```python
from build123d import *

# Parameters (mm, degrees)
F2_DEPTH = 10.16
F3_R     = 2.413
F4_DEPTH = 10.16
F5_R     = 5.08
F6_R     = 1.27
F8_DEPTH = 10.16
F9_R     = 5.08


# Not quite as in the source:
# - a variable given as a bare number and used for a length is read in inches; the dataset says mm whatever the document's units were
# - a feature names something its author has since deleted; it is built from what else it names


with BuildPart() as f2:
    # F1 (on Top) → F2 (new body)
    with BuildSketch(Plane.XY):
        with BuildLine():
            Line((0, 0), (0, -76.2))
            Line((0, -76.2), (0, -82.55))
            ThreePointArc((0, -82.55), (4.4901280605, -80.6901280605), (6.35, -76.2))
            Line((6.35, -76.2), (6.35, 5.1130828846))
            ThreePointArc((6.35, 5.1130828846), (-16.8661271179, 9.1115403998), (-40.386, 10.4501219109))
            ThreePointArc((-40.386, 10.4501219109), (-63.9058728821, 9.1115403998), (-87.122, 5.1130828846))
            Line((-87.122, 5.1130828846), (-87.122, -76.2))
            ThreePointArc((-87.122, -76.2), (-85.2621280605, -80.6901280605), (-80.772, -82.55))
            Line((-80.772, -82.55), (-80.772, -76.2))
            Line((-80.772, -76.2), (-80.772, 0))
            ThreePointArc((-80.772, 0), (-60.6827977504, 3.072463713), (-40.386, 4.1001219109))
            ThreePointArc((-40.386, 4.1001219109), (-20.0892022496, 3.072463713), (0, 0))
        make_face()
    extrude(amount=F2_DEPTH)

    # F3 (on Top) → F4 (join)
    with BuildSketch(Plane.XY):
        with Locations((0, -7.9375)):
            Circle(F3_R)
        with Locations((-80.772, -7.9375)):
            Circle(F3_R)
    extrude(amount=F4_DEPTH)

    # F5
    f5_edges = [f2.edges().sort_by_distance(p)[0] for p in [
        (-87.122, 5.113083, 5.08),
        (6.35, 5.113083, 5.08),
    ]]
    fillet(f5_edges, radius=F5_R)

    # F6
    f6_edges = [f2.edges().sort_by_distance(p)[0] for p in [
        (0, -82.55, 5.08),
        (-80.772, -82.55, 5.08),
        (0, 0, 5.08),
        (-80.772, 0, 5.08),
    ]]
    fillet(f6_edges, radius=F6_R)

    # F7 (on Top) → F8 (join)
    with BuildSketch(Plane.XY):
        with BuildLine():
            ThreePointArc((31.75, -25.4), (19.05, -38.1), (6.35, -25.4))
            Line((6.35, -25.4), (6.35, -65.42595876))
            ThreePointArc((6.35, -65.42595876), (11.6697145424, -58.7651555547), (19.05, -54.499355663))
            ThreePointArc((19.05, -54.499355663), (32.9139558425, -42.7901912008), (38.1, -25.4))
            ThreePointArc((38.1, -25.4), (34.925, -28.575), (31.75, -25.4))
        make_face()
        with BuildLine():
            ThreePointArc((38.1, -25.4), (34.925, -22.225), (31.75, -25.4))
            ThreePointArc((31.75, -25.4), (34.925, -28.575), (38.1, -25.4))
        make_face()
        with BuildLine():
            Line((-87.122, -65.42595876), (-87.122, -25.4))
            ThreePointArc((-87.122, -25.4), (-99.822, -38.1), (-112.522, -25.4))
            ThreePointArc((-112.522, -25.4), (-115.697, -28.575), (-118.872, -25.4))
            ThreePointArc((-118.872, -25.4), (-113.6859558425, -42.7901912008), (-99.822, -54.499355663))
            ThreePointArc((-99.822, -54.499355663), (-92.4417145424, -58.7651555547), (-87.122, -65.42595876))
        make_face()
        with BuildLine():
            ThreePointArc((-118.872, -25.4), (-115.697, -28.575), (-112.522, -25.4))
            ThreePointArc((-112.522, -25.4), (-115.697, -22.225), (-118.872, -25.4))
        make_face()
    extrude(amount=F8_DEPTH)

    # F9
    f9_edges = [f2.edges().sort_by_distance(p)[0] for p in [
        (6.35, -65.425959, 5.08),
        (-87.122, -65.425959, 5.08),
    ]]
    fillet(f9_edges, radius=F9_R)


solid = f2.part
```
The model under review builds one solid part; all positions refer to its coordinate system, in mm. A direction names the side the tool comes from. Round coordinates to 2 decimals unless told otherwise and drop trailing zeros. Write each loop counter-clockwise with the first axis right and the second up, starting at its lowest first coordinate (ties: lowest second). Pieces come first, ordered by that corner, then holes. Notation, with made-up numbers: M -10,47.5 L 9,47.5 A36 ccw 9,85.5 Z; hole C 74.25,30 d6. An arc over 180 degrees is marked long. Use CSV: the item, a comma, the result in double quotes. Start each with the question number.
(1) We need section C-C, the plane x = -54.5. State the section outline as (y, z) points, then the cut area to 3 significant figures.
(2) We need section A-A, the plane y = -47. State the section outline as (x, z) points, then the cut area to 3 significant figures.
(3) Tool access review of faces 1 (the face through (-80.772, -46, 5)), 2 (the face through (-47, 6, 10.16)), 3 (the face through (-80.772, -3, 5)): name each direction out of +Z, -Z, +X, -X, +Y, -Y from which nothing blocks a thin tool from reaching the whole face with its end or side.
(4) For line 1 along X through (y, z) = (-74, 6.5); line 2 along X through (y, z) = (-35.5, 9), list the stretches that pass through material, from the lowest coordinate up.
(5) The part is to be moulded in two halves that separate along Y. For faces 4 (the face through (34.995, -22.226, 5.009)), 5 (the face through (6.35, -72, 5)), 6 (the face through (0, -3, 5)), say which applies: +Y half, -Y half, draft (parallel to the pull), parting line (faces both ways), or undercut.
(6) Clearance check with flat-ended pins moving along their axes: P1, Ø3, axis at x = -35, z = 8.5, coming from the -Y side; P2, Ø6, axis at x = -20, z = 7.5, coming from the -Y side; P3, Ø2, axis at y = -3, z = 6.5, coming from the +X side. State where each tip first meets the part, or that it passes through.
Findings:
1,outline,"M 3.6,0 L 9.97,0 L 9.97,10.16 L 3.6,10.16 Z"
1,area,"64.7 mm^2"
2,outline,"M -110.39,0 L -80.77,0 L -80.77,10.16 L -110.39,10.16 Z; M 0,0 L 29.62,0 L 29.62,10.16 L 0,10.16 Z"
2,area,"602 mm^2"
3,face 1,"+Z, -Z, -Y"
3,face 2,"+Z, +X, -X, +Y, -Y"
3,face 3,"+Z, -Z"
4,line 1,"-87.12 to -80.77, 0 to 6.35"
4,line 2,"-117.22 to -107.52, -92.12 to -80.77, 0 to 11.35, 26.75 to 36.45"
5,face 4,"+Y half"
5,face 5,"draft"
5,face 6,"undercut"
6,P1,"y = 3.98"
6,P2,"y = 2.73"
6,P3,"x = 6.35"
